Answer from the drawing. Dimensions are ordinates in mm from the lowest x, y and z of the part. A direction names the side the tool comes from. Give positions to 0.01 mm unless a question says otherwise; leave off trailing zeros. Loops run counter-clockwise (first coordinate to the right, second up) from the corner with the lowest first, then second, coordinate; pieces in that order, holes last.
Item 1: Each of these flat-tipped pins is pushed along its axis until it touches: pin 1 Ø1.5 at (y, z) = (7.5, 3) entering from -X; pin 2 Ø0.8 at (x, y) = (35, 14) entering from -Z; pin 3 Ø2.5 at (x, z) = (1.5, 5) entering from +Y; pin 4 Ø5 at (x, z) = (8.5, 5) entering from +Y. Where does it stop, or does it pass through?
Item 2: A tool of negligible diameter and unlimited length cuts with its end or side. For the marked faces 1, 2 and 3, from which of +Z, -Z, +X, -X, +Y, -Y can it reach the whole face along a straight path? Write none if from no direction.
Item 3: Section B-B, the plane z = 6.75 is taken. Give the vertices of the cut face in (x, y), and give its area (4 significant figures).
Item 4: Consider line 1 along X through (y, z) = (7.75, 5); line 2 along Y through (x, z) = (10, 6.25); line 3 along X through (y, z) = (26.75, 4.25). Determine where each line is inside the solid, lowest interval first.
Item 5: The mould has two halves that part along Z. Classify the marked faces 4, 5 and 6: pulls with the +Z half, pulls with the -Z half, needs draft (parallel to the pull), parting line crosses it, or undercut.
Item 6: Section D-D, the plane y = 18.75 is taken. Give the vertices of the cut face in (x, z), and give its area (3 significant figures).
Item 7: Section A-A, the plane y = 15.5 is taken. Give the vertices of the cut face in (x, z), and give its area (3 significant figures).
Item 8: Section C-C, the plane z = 2 is taken. Give the vertices of the cut face in (x, y).
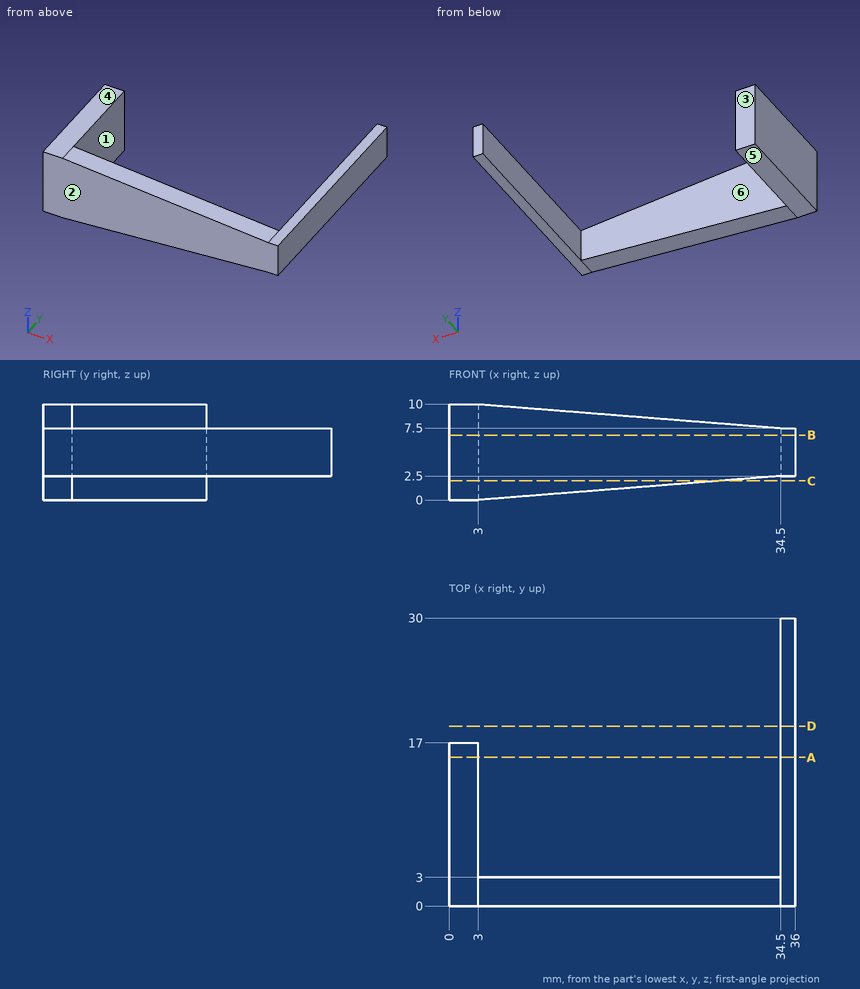
Worked answers:
1. pin 1: stops at x = 0
1. pin 2: stops at z = 2.5
1. pin 3: stops at y = 17
1. pin 4: stops at y = 3
2. face 1: +Z, -Z, +Y
2. face 2: +Z, -Z, +X, -X, -Y
2. face 3: +Z, -Z, -X, +Y
3. outline: (0, 0) - (36, 0) - (36, 30) - (34.5, 30) - (34.5, 3) - (3, 3) - (3, 17) - (0, 17) - close
3. area: 190.5 mm2
4. line 1: x = 0 to 3, 34.5 to 36
4. line 2: y = 0 to 3
4. line 3: x = 34.5 to 36
5. face 4: pulls with the +Z half
5. face 5: pulls with the -Z half
5. face 6: needs draft
6. outline: (34.5, 2.5) - (36, 2.5) - (36, 7.5) - (34.5, 7.5) - close
6. area: 7.50 mm2
7. outline: (0, 0) - (3, 0) - (3, 10) - (0, 10) - close; (34.5, 2.5) - (36, 2.5) - (36, 7.5) - (34.5, 7.5) - close
7. area: 37.5 mm2
8. outline: (0, 0) - (28.2, 0) - (28.2, 3) - (3, 3) - (3, 17) - (0, 17) - close
